from build123d import *

# Parameters (mm, degrees)
F0_R      = 51
F1_DEPTH  = 42.5
F2_R      = 17.5
F3_R      = 24.5
F4_DEPTH  = 17.8
F5_R      = 1
F6_DEPTH  = 42.5
F7_R      = 33
F8_DEPTH  = 11
F9_R      = 24.5
F10_DEPTH = 80
F11_R     = 17.5
F17_ANGLE = 180
F19_R     = 7.6099640243
F20_DEPTH = 7
F21_R     = 24.25
F22_DEPTH = 80


with BuildPart() as f1:
    # F0 (on Top) → F1 (new body)
    with BuildSketch(Plane.XY):
        Circle(F0_R)
    extrude(amount=F1_DEPTH)

    # F2
    f2_edges = [f1.edges().sort_by_distance(p)[0] for p in [
        (-51, 0, 42.5),
    ]]
    fillet(f2_edges, radius=F2_R)

    # F3 (on face) → F4 (join)
    with BuildSketch(Plane.XY.offset(42.5)):
        Circle(F3_R)
    extrude(amount=F4_DEPTH)

    # F5
    f5_edges = [f1.edges().sort_by_distance(p)[0] for p in [
        (-24.5, 0, 60.3),
    ]]
    fillet(f5_edges, radius=F5_R)

    # F6 (add): a face of the model
    f6_faces = [f1.faces().sort_by_distance(p)[0] for p in [
        (0, 0, 0),
    ]]
    extrude(f6_faces, amount=F6_DEPTH)

    # F7 (on face) → F8 (join)
    with BuildSketch(Plane(origin=(0, 0, -42.5), x_dir=(1, 0, 0), z_dir=(0, 0, -1))):
        Circle(F7_R)
    extrude(amount=F8_DEPTH)

    # F9 (on face) → F10 (cut)
    with BuildSketch(Plane(origin=(0, 0, -53.5), x_dir=(1, 0, 0), z_dir=(0, 0, -1))):
        Circle(F9_R)
    extrude(amount=-F10_DEPTH, mode=Mode.SUBTRACT)

    # F11
    f11_edges = [f1.edges().sort_by_distance(p)[0] for p in [
        (-51, 0, -42.5),
    ]]
    fillet(f11_edges, radius=F11_R)

    # F16 (on offset) → F17 (revolve, cut)
    with BuildSketch(Plane.XZ.offset(25)):
        with BuildLine():
            Line((35, 0), (45, 0))
            ThreePointArc((45, 0), (0, 32.271534479), (-45, 0))
            Line((-45, 0), (-35, 0))
            ThreePointArc((-35, 0), (0, 15.7988658705), (35, 0))
        make_face()
    revolve(axis=Axis((0, -25, 0), (1, 0, 0)), revolution_arc=F17_ANGLE, mode=Mode.SUBTRACT)


with BuildPart() as f14:
    # F13 (on offset) → F14 (revolve)
    with BuildSketch(Plane.XZ.offset(25)):
        with BuildLine():
            Line((-35, 0), (35, 0))
            ThreePointArc((35, 0), (0, 15.4876255188), (-35, 0))
        make_face()
    revolve(axis=Axis((0, -25, 0), (1, 0, 0)))


with BuildPart() as f20_tool:
    # F19 (on offset) → F20 (new body)
    with BuildSketch(Plane.XZ.offset(45)):
        Circle(F19_R)
    extrude(amount=-F20_DEPTH)


with BuildPart() as f1_1:
    add(f1.part)

    # F20: cut by f20_tool
    add(f20_tool.part, mode=Mode.SUBTRACT)


with BuildPart() as f14_1:
    add(f14.part)

    # F20: cut by f20_tool
    add(f20_tool.part, mode=Mode.SUBTRACT)

    # F21 (on face) → F22 (cut)
    with BuildSketch(Plane(origin=(0, 0, -53.5), x_dir=(1, 0, 0), z_dir=(0, 0, -1))):
        Circle(F21_R)
    extrude(amount=-F22_DEPTH, mode=Mode.SUBTRACT)


solid = f1_1.part
Design review of the part built by this model. Coordinates are the model's own, in mm. A direction names the side the tool comes from. Round coordinates to 2 decimals unless told otherwise and drop trailing zeros. Write each loop counter-clockwise with the first axis right and the second up, starting at its lowest first coordinate (ties: lowest second). Pieces come first, ordered by that corner, then holes. Notation, with made-up numbers: (6, 33.25) - (46, 33.25) arc R13 ccw to (46, 58.25) - close; hole circle Ø4 at (10, -17). An arc over 180 degrees is marked (long way). Use a Markdown table: item, result. Add a question column.
1. Mouldability with a two-part tool opening along Z and no side actions: class faces 6 (the face through (2, -25, 42.5)), 7 (the face through (-1.65, -38.62, -7.43)), 8 (the face through (0, -25, -53.5)) as +Z half, -Z half, draft (parallel to the pull), parting line (faces both ways), or undercut.
2. We need section A-A (y = 0). State the section outline as (x, z) points, then the cut area to 3 significant figures.
3. Clearance check with flat-ended pins moving along their axes: pin 1 (5 mm diameter, centred on y = 18.5, z = 10.5, fed in from -X); pin 2 (8 mm diameter, centred on y = 7, z = 29, fed in from +X); pin 3 (20 mm diameter, centred on x = -15, y = -12, fed in from -Z); pin 4 (4.5 mm diameter, centred on x = 2.5, z = 2.5, fed in from -Y). State where each tip first meets the part, or that it passes through.
4. Wall thickness on probe 1 along X at (y, z) = (-26, 8.5); probe 2 along X at (y, z) = (-1, -25); probe 3 along Z at (x, y) = (32.5, -26): over which ranges is each line inside the solid? List them lowest first.
5. We need section B-B (z = 37). State the section outline as (x, y) points.
6. For faces 1 (the face through (13.17, 20.66, 50.78)), 2 (the face through (0, 0, 60.3)), 3 (the face through (-11, -25, -15)), 4 (the face through (0, -38, 0)), 5 (the face through (0, 0, 26.5)), list the 3-axis set-ups (+Z, -Z, +X, -X, +Y, -Y) from which the entire face can be reached by the end or side of a thin tool; tool diameter is ignored.
Output:
| question | item | result |
|---|---|---|
| 1 | face 6 | +Z half |
| 1 | face 7 | undercut |
| 1 | face 8 | -Z half |
| 2 | outline | (-51, -25) arc R17.5 ccw to (-33.5, -42.5) - (-33, -42.5) - (-33, -53.5) - (-24.5, -53.5) - (-24.5, 26.5) - (24.5, 26.5) - (24.5, -53.5) - (33, -53.5) - (33, -42.5) - (33.5, -42.5) arc R17.5 ccw to (51, -25) - (51, 25) arc R17.5 ccw to (33.5, 42.5) - (24.5, 42.5) - (24.5, 59.3) arc R1 ccw to (23.5, 60.3) - (-23.5, 60.3) arc R1 ccw to (-24.5, 59.3) - (-24.5, 42.5) - (-33.5, 42.5) arc R17.5 ccw to (-51, 25) - close |
| 2 | area | 6,080 mm2 |
| 3 | pin 1 | stops at x = -48.43 |
| 3 | pin 2 | stops at x = 50.79 |
| 3 | pin 3 | stops at z = -53.5 |
| 3 | pin 4 | stops at y = -38 |
| 4 | probe 1 | x = -43.87 to -41.12, -24.97 to 24.97, 41.12 to 43.87 |
| 4 | probe 2 | x = -50.99 to -24.48, 24.48 to 50.99 |
| 4 | probe 3 | z = -40.5 to -19.39, -2.42 to 2.42, 19.39 to 40.5 |
| 5 | outline | circle Ø92.48 at (0, 0) |
| 6 | face 1 | +Z |
| 6 | face 2 | +Z, +X, -X, +Y, -Y |
| 6 | face 3 | none |
| 6 | face 4 | -Y |
| 6 | face 5 | -Z |
